Verification items for the finished model (mm, model axes). Give positions to 0.01 mm unless a question says otherwise; leave off trailing zeros. Loops run counter-clockwise (first coordinate to the right, second up) from the corner with the lowest first, then second, coordinate; pieces in that order, holes last. Notation, with made-up numbers: M 45.25,20 L 56.25,20 A9 cw 56.25,26 Z; hole C 24,5 d11. An arc over 180 degrees is marked long. Use CSV: the item, a comma, the result in double quotes.
from build123d import *

# Parameters (mm, degrees)
F0_R     = 28.5
F0_R_2   = 17
F1_DEPTH = 2.5
F3_DEPTH = 25
F6_DEPTH = 25
F7_DEPTH = 25


with BuildPart() as f1:
    # F0 (on Front) → F1 (new body)
    with BuildSketch(Plane.XZ):
        Circle(F0_R)
        Circle(F0_R_2, mode=Mode.SUBTRACT)
    extrude(amount=F1_DEPTH)

    # F2 (on face) → F3 (cut)
    with BuildSketch(Plane.XZ.offset(2.5)):
        with BuildLine():
            Line((-25.75, 0), (-19.75, 0))
            ThreePointArc((-19.75, 0), (-22.75, 3), (-25.75, 0))
        make_face()
        with BuildLine():
            ThreePointArc((-25.75, 0), (-22.75, -3), (-19.75, 0))
            Line((-19.75, 0), (-25.75, 0))
        make_face()
        with BuildLine():
            ThreePointArc((25.75, 0), (22.75, 3), (19.75, 0))
            Line((19.75, 0), (25.75, 0))
        make_face()
        with BuildLine():
            Line((25.75, 0), (19.75, 0))
            ThreePointArc((19.75, 0), (22.75, -3), (25.75, 0))
        make_face()
    extrude(amount=-F3_DEPTH, mode=Mode.SUBTRACT)

    # F5 (on face) → F6 (cut)
    with BuildSketch(Plane.XZ.offset(2.5)):
        with BuildLine():
            Line((-24.75, 7), (-22.75, 7))
            Line((-22.75, 7), (-20.75, 7))
            ThreePointArc((-20.75, 7), (-22.75, 9), (-24.75, 7))
        make_face()
        with BuildLine():
            Line((-22.75, 7), (-22.75, 5))
            ThreePointArc((-22.75, 5), (-21.3357864376, 5.5857864376), (-20.75, 7))
            Line((-20.75, 7), (-22.75, 7))
        make_face()
        with BuildLine():
            ThreePointArc((-24.75, 7), (-24.1642135624, 5.5857864376), (-22.75, 5))
            Line((-22.75, 5), (-22.75, 7))
            Line((-22.75, 7), (-24.75, 7))
        make_face()
    extrude(amount=-F6_DEPTH, mode=Mode.SUBTRACT)

    # F4 (on face) → F7 (cut)
    with BuildSketch(Plane.XZ.offset(2.5)):
        with BuildLine():
            Line((24.75, -7), (22.75, -7))
            Line((22.75, -7), (20.75, -7))
            ThreePointArc((20.75, -7), (22.75, -9), (24.75, -7))
        make_face()
        with BuildLine():
            Line((22.75, -7), (22.75, -5))
            ThreePointArc((22.75, -5), (21.3357864376, -5.5857864376), (20.75, -7))
            Line((20.75, -7), (22.75, -7))
        make_face()
        with BuildLine():
            ThreePointArc((24.75, -7), (24.1642135624, -5.5857864376), (22.75, -5))
            Line((22.75, -5), (22.75, -7))
            Line((22.75, -7), (24.75, -7))
        make_face()
    extrude(amount=-F7_DEPTH, mode=Mode.SUBTRACT)


solid = f1.part
(1) Section check C-C on z = -10. Record the cut outline in (x, y), plus the area to 3 significant figures.
Calculated:
outline,"M -26.69,-2.5 L -13.75,-2.5 L -13.75,0 L -26.69,0 Z; M 13.75,-2.5 L 26.69,-2.5 L 26.69,0 L 13.75,0 Z"
area,"64.7 mm²"
(2) Section check A-A on x = 0. Record the cut outline in (y, z), plus the area to 3 significant figures.
Calculated:
outline,"M -2.5,-28.5 L 0,-28.5 L 0,-17 L -2.5,-17 Z; M -2.5,17 L 0,17 L 0,28.5 L -2.5,28.5 Z"
area,"57.5 mm²"
(3) Section check D-D on z = 8. Record the cut outline in (x, y), plus the area to 3 significant figures.
Calculated:
outline,"M -27.35,-2.5 L -24.48,-2.5 L -24.48,0 L -27.35,0 Z; M -21.02,-2.5 L -15,-2.5 L -15,0 L -21.02,0 Z; M 15,-2.5 L 27.35,-2.5 L 27.35,0 L 15,0 Z"
area,"53.1 mm²"
(4) Section check B-B on y = -1.1. Record the cut outline in (x, z).
Calculated:
outline,"C 0,0 d57; hole C -22.75,0 d6; hole C -22.75,7 d4; hole C 0,0 d34; hole C 22.75,0 d6; hole C 22.75,-7 d4"
(5) Depth check by flat-ended pin: pin 1 Ø1.5 at (x, y) = (21.5, -1) entering from -Z; pin 2 Ø1 at (x, y) = (22, -0.5) entering from -Z; pin 3 Ø1 at (y, z) = (-1.5, -22) entering from +X; pin 4 Ø5 at (x, z) = (-22.75, 0) entering from -Y. Enter the tip coordinate at first touch or a pass-through.
Calculated:
pin 1,"stops at z = -19.54"
pin 2,"stops at z = -18.71"
pin 3,"stops at x = 18.71"
pin 4,"passes through"
(6) Mould release check, pull along X, two halves, no side actions. Record for faces 1 (the cylindrical face through (26.327, -1.232, -10.916)), 2 (the flat face through (12.3, -2.5, -12.3)), 3 (the cylindrical face through (25.747, -1.268, -0.132)): released by +X, released by -X, zero draft, split by the parting line, or undercut.
Calculated:
face 1,"split by the parting line"
face 2,"zero draft"
face 3,"undercut"
(7) Scan lines: L1, parallel to Z at x = -21.5, y = -1.6; L2, parallel to Z at x = 22.75, y = -1.15; L3, parallel to Z at x = 0.5, y = -2.35. Record each from-to range of solid material in increasing order. Write a range as from..to.
Calculated:
L1,"z = -18.71..-2.73, 2.73..5.44, 8.56..18.71"
L2,"z = -17.17..-9, -5..-3, 3..17.17"
L3,"z = -28.5..-16.99, 16.99..28.5"
